Autodesk Inventor part; units mm, degrees
ref_plane "YZ Plane" through (0, 0, 0) normal (1, 0, 0) x (0, 1, 0)
ref_plane "XZ Plane" through (0, 0, 0) normal (0, 1, 0) x (-1, 0, 0)
ref_plane "XY Plane" through (0, 0, 0) normal (0, 0, 1) x (1, 0, 0)
sketch "Sketch1" plane through (0, 0, 0) normal (0, 0, 1) x (1, 0, 0)
  arc A0 (219.754, -304.8) -> (225.7704, -296.4188) centre (219.754, -298.45) ccw
  line L0 (225.7704, -296.4188) -> (30.0819, 283.206)
  arc A1 (30.0819, 283.206) -> (-30.0819, 283.206) centre (0, 273.05) ccw
  line L1 (-30.0819, 283.206) -> (-225.7704, -296.4188)
  arc A2 (-225.7704, -296.4188) -> (-219.754, -304.8) centre (-219.754, -298.45) ccw
  line L2 (-219.754, -304.8) -> (219.754, -304.8)
  line L3 (-38.1, -17.4222) -> (-38.1, -222.25)
  arc A3 (-44.45, -228.6) -> (-38.1, -222.25) centre (-44.45, -222.25) ccw
  line L4 (-44.45, -228.6) -> (-113.6024, -228.6)
  arc A4 (-119.6188, -220.2188) -> (-113.6024, -228.6) centre (-113.6024, -222.25) ccw
  line L5 (-119.6188, -220.2188) -> (-50.4664, -15.391)
  arc A5 (-38.1, -17.4222) -> (-50.4664, -15.391) centre (-44.45, -17.4222) ccw
  line L6 (113.6024, -228.6) -> (44.45, -228.6)
  arc A6 (38.1, -222.25) -> (44.45, -228.6) centre (44.45, -222.25) ccw
  line L7 (38.1, -222.25) -> (38.1, -17.4222)
  arc A7 (50.4664, -15.391) -> (38.1, -17.4222) centre (44.45, -17.4222) ccw
  line L8 (50.4664, -15.391) -> (119.6188, -220.2188)
  arc A8 (113.6024, -228.6) -> (119.6188, -220.2188) centre (113.6024, -222.25) ccw
  circle A9 centre (-204.2059, -292.1) radius 2
  circle A10 centre (-187.0552, -241.3) radius 2
  circle A11 centre (187.0552, -241.3) radius 2
  circle A12 centre (204.2059, -292.1) radius 2
  circle A13 centre (19.05, -241.3) radius 2
  circle A14 centre (19.05, -292.1) radius 2
  circle A15 centre (-19.05, -292.1) radius 2
  circle A16 centre (-19.05, -241.3) radius 2
  circle A17 centre (8.89, 288.4479) radius 2
  circle A18 centre (-8.89, 288.4479) radius 2
  circle A19 centre (-17.78, 273.05) radius 2
  circle A20 centre (-8.89, 257.6521) radius 2
  circle A21 centre (8.89, 257.6521) radius 2
  circle A22 centre (17.78, 273.05) radius 2
  circle A23 centre (0, 273.05) radius 11.0762
  circle A24 centre (0, 273.05) radius 20.955
  circle A25 centre (-8.89, 288.4479) radius 2.1
  circle A26 centre (8.89, 288.4479) radius 2.1
  circle A27 centre (17.78, 273.05) radius 2.1
  circle A28 centre (8.89, 257.6521) radius 2.1
  circle A29 centre (-8.89, 257.6521) radius 2.1
  circle A30 centre (-17.78, 273.05) radius 2.1
  ellipse E0 centre (0, 273.05) end of major axis (-12.7, 273.05) minor radius 12.2673
  point P0 (0, 0)
  dimension "d1" = 41.91
  dimension "d2" = 4.2
  dimension "d3" = 4.2
  dimension "d4" = 4.2
  dimension "d5" = 4.2
  dimension "d6" = 4.2
  dimension "d7" = 4.2
extrude "Extrusion1" add sketch "Sketch1" along normal blind 3.175 contours A24 | E0
chamfer "Chamfer1" distance 0.635 angle 45 7 edges at (-11.0762, 273.05, 0) (-10.99, 288.4479, 3.175) (-19.88, 273.05, 3.175) (-10.99, 257.6521, 3.175) (6.79, 257.6521, 3.175) (15.68, 273.05, 3.175) (6.79, 288.4479, 3.175)
properties part number "MainInnerBearingMount"
Model file for the job. Use its own axes, mm. Give positions to 0.01 mm unless a question says otherwise; leave off trailing zeros. Write each loop counter-clockwise with the first axis right and the second up, starting at its lowest first coordinate (ties: lowest second). Pieces come first, ordered by that corner, then holes. Notation, with made-up numbers: M -4.75,6.25 L 33.25,6.25 A20 ccw 33.25,30.25 Z; hole C 70,81.5 d3. An arc over 180 degrees is marked long. One line per item, written item: value. Start each with the question number.
Q1. Two-plate mould, pull along Y, no slides. Class faces 1 (the flat face through (9, 264, 0)), 2 (the cylindrical face through (-9.163, 286.366, 1.252)), 3 (the cylindrical face through (-4.543, 293.507, 1.565)): +Y half, -Y half, draft (parallel to the pull), parting line (faces both ways), or undercut.
Q2. Drop flat-ended pins along their axis: pin 1 Ø1.5 at (y, z) = (285.5, 2.5) entering from +X; pin 2 Ø1.5 at (y, z) = (269, 1.5) entering from -X; pin 3 Ø1 at (x, z) = (-5.5, 2) entering from -Y. Give the stop position or say it passes through.
Q3. Probe probe 1 along X at (y, z) = (272.5, 1.5); probe 2 along Y at (x, z) = (17.78, 1.35); probe 3 along X at (y, z) = (271.5, 2.65). List the from-to ranges inside material, lowest first. Write a range as [from, to].
Q4. Saw through at A-A, the plane y = 273.05. Write the cut outline in (x, z) (3 decimals), plus the area to 3 significant figures.
Q5. Saw through at B-B, the plane x = 0. Write the cut outline in (y, z) (3 decimals), plus the area to 3 significant figures.
Q6. Saw through at D-D, the plane y = 287.5. State how many separate pieces and enclosed holes the cut face has, plus the area to 3 significant figures.
Q7. Saw through at C-C, the plane z = 1.25. Write the cut outline in (x, y) (3 decimals), plus the area to 3 significant figures.
Output values:
1. face 1: draft
1. face 2: undercut
1. face 3: parting line
2. pin 1: stops at x = 17.38
2. pin 2: stops at x = -20.69
2. pin 3: stops at y = 252.7
3. probe 1: x = [-20.95, -19.81], [-15.75, -11.06], [11.06, 15.75], [19.81, 20.95]
3. probe 2: y = [261.96, 270.95], [275.15, 284.14]
3. probe 3: x = [-20.9, -19.36], [-16.2, -10.97], [10.97, 16.2], [19.36, 20.9]
4. outline: M -20.955,0 L -19.88,0 L -19.88,2.54 L -20.515,3.175 L -20.955,3.175 Z; M -15.68,0 L -11.711,0 L -11.076,0.635 L -11.076,3.175 L -15.045,3.175 L -15.68,2.54 Z; M 11.076,0.635 L 11.711,0 L 15.68,0 L 15.68,2.54 L 15.045,3.175 L 11.076,3.175 Z; M 19.88,0 L 20.955,0 L 20.955,3.175 L 20.515,3.175 L 19.88,2.54 Z
4. area: 34.9 mm²
5. outline: M 252.095,0 L 261.339,0 L 261.974,0.635 L 261.974,3.175 L 252.095,3.175 Z; M 284.126,0.635 L 284.761,0 L 294.005,0 L 294.005,3.175 L 284.126,3.175 Z
5. area: 62.3 mm²
6. separate pieces: 3
6. enclosed holes: 0
6. area: 71.7 mm²
7. outline: C 0,273.05 d41.91; hole C -17.78,273.05 d4.2; hole C 0,273.05 d22.152; hole C -8.89,257.652 d4.2; hole C -8.89,288.448 d4.2; hole C 8.89,257.652 d4.2; hole C 8.89,288.448 d4.2; hole C 17.78,273.05 d4.2
7. area: 911 mm²
